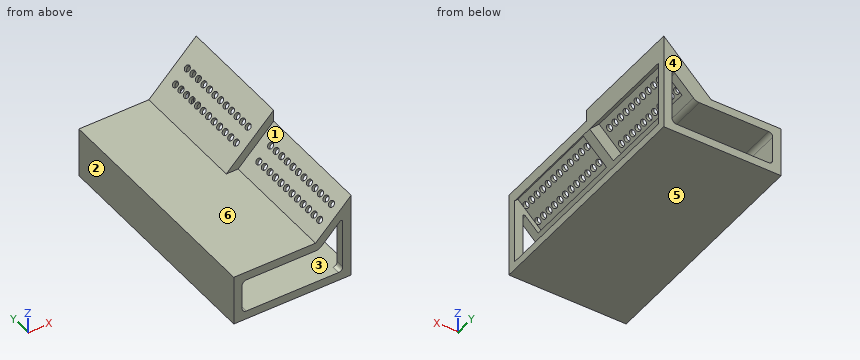
from build123d import *

# Parameters (mm, degrees)
F1_DEPTH  = 70
F3_DEPTH  = 65
F5_DEPTH  = 70
F6_R      = 2.5
F7_R      = 5
F8_R      = 1
F9_R      = 1.875
F10_DEPTH = 41.214203
F11_W     = 61.875
F11_H     = 20
F12_DEPTH = 3
F13_R     = 1.875
F14_DEPTH = 8


with BuildPart() as f1:
    # F0 (on Front) → F1 (new body, symmetric)
    with BuildSketch(Plane.XZ):
        Polygon((-35, 30), (-35, 0), (35, 0), (35, 30), (35, 51.213203), (13.786797, 30), align=None)
        Polygon((30, 5), (-30, 5), (-30, 25), (15.857864, 25), (30, 39.142136), (30, 30), align=None, mode=Mode.SUBTRACT)
    extrude(amount=F1_DEPTH, both=True)

    # F2 (on Front) → F3 (cut, symmetric)
    with BuildSketch(Plane.XZ):
        Polygon((35, 44.142136), (30, 39.142136), (30, 5), (35, 5), align=None)
    extrude(amount=F3_DEPTH, both=True, mode=Mode.SUBTRACT)

    # F4 (on face) → F5 (join)
    with BuildSketch(Plane(origin=(0, 70, 0), x_dir=(-1, 0, 0), z_dir=(0, 1, 0))):
        Polygon((-13.786797, 30), (-6.715729, 30), (-35, 58.284271), (-35, 51.213203), align=None)
    extrude(amount=-F5_DEPTH)

    # F6
    f6_edges = [f1.edges().sort_by_distance(p)[0] for p in [
        (-30, 0, 5),
        (-30, 0, 25),
        (30, 67.5, 5),
        (30, -67.5, 5),
    ]]
    fillet(f6_edges, radius=F6_R)

    # F7
    f7_edges = [f1.edges().sort_by_distance(p)[0] for p in [
        (15.857864, 0, 25),
    ]]
    fillet(f7_edges, radius=F7_R)

    # F8
    f8_edges = [f1.edges().sort_by_distance(p)[0] for p in [
        (30, 67.5, 39.142136),
        (30, -67.5, 39.142136),
    ]]
    fillet(f8_edges, radius=F8_R)

    # F9 (on face) → F10 (cut, through all)
    with BuildSketch(Plane(origin=(-11.642136, 0, 11.642136), x_dir=(0, -1, 0), z_dir=(-0.707107, 0, 0.707107))):
        with Locations((-62, 50.961941)):
            Circle(F9_R)
        with Locations((-57, 50.961941)):
            Circle(F9_R)
        with Locations((-52, 50.961941)):
            Circle(F9_R)
        with Locations((-47, 50.961941)):
            Circle(F9_R)
        with Locations((-42, 50.961941)):
            Circle(F9_R)
        with Locations((-37, 50.961941)):
            Circle(F9_R)
        with Locations((-32, 50.961941)):
            Circle(F9_R)
        with Locations((-27, 50.961941)):
            Circle(F9_R)
        with Locations((-22, 50.961941)):
            Circle(F9_R)
        with Locations((-17, 50.961941)):
            Circle(F9_R)
        with Locations((-12, 50.961941)):
            Circle(F9_R)
        with Locations((-7, 50.961941)):
            Circle(F9_R)
        with Locations((8, 50.961941)):
            Circle(F9_R)
        with Locations((13, 50.961941)):
            Circle(F9_R)
        with Locations((18, 50.961941)):
            Circle(F9_R)
        with Locations((23, 50.961941)):
            Circle(F9_R)
        with Locations((28, 50.961941)):
            Circle(F9_R)
        with Locations((33, 50.961941)):
            Circle(F9_R)
        with Locations((38, 50.961941)):
            Circle(F9_R)
        with Locations((43, 50.961941)):
            Circle(F9_R)
        with Locations((48, 50.961941)):
            Circle(F9_R)
        with Locations((53, 50.961941)):
            Circle(F9_R)
        with Locations((58, 50.961941)):
            Circle(F9_R)
        with Locations((63, 50.961941)):
            Circle(F9_R)
        with Locations((-62, 40.961941)):
            Circle(F9_R)
        with Locations((-57, 40.961941)):
            Circle(F9_R)
        with Locations((-52, 40.961941)):
            Circle(F9_R)
        with Locations((-47, 40.961941)):
            Circle(F9_R)
        with Locations((-42, 40.961941)):
            Circle(F9_R)
        with Locations((-37, 40.961941)):
            Circle(F9_R)
        with Locations((-32, 40.961941)):
            Circle(F9_R)
        with Locations((-27, 40.961941)):
            Circle(F9_R)
        with Locations((-22, 40.961941)):
            Circle(F9_R)
        with Locations((-17, 40.961941)):
            Circle(F9_R)
        with Locations((-12, 40.961941)):
            Circle(F9_R)
        with Locations((-7, 40.961941)):
            Circle(F9_R)
        with Locations((8, 40.961941)):
            Circle(F9_R)
        with Locations((13, 40.961941)):
            Circle(F9_R)
        with Locations((18, 40.961941)):
            Circle(F9_R)
        with Locations((23, 40.961941)):
            Circle(F9_R)
        with Locations((28, 40.961941)):
            Circle(F9_R)
        with Locations((33, 40.961941)):
            Circle(F9_R)
        with Locations((38, 40.961941)):
            Circle(F9_R)
        with Locations((43, 40.961941)):
            Circle(F9_R)
        with Locations((48, 40.961941)):
            Circle(F9_R)
        with Locations((53, 40.961941)):
            Circle(F9_R)
        with Locations((58, 40.961941)):
            Circle(F9_R)
        with Locations((63, 40.961941)):
            Circle(F9_R)
    extrude(amount=-F10_DEPTH, mode=Mode.SUBTRACT)

    # F11 (on face) → F12 (cut)
    with BuildSketch(Plane(origin=(-4.571068, 0, 4.571068), x_dir=(0, 1, 0), z_dir=(0.707107, 0, -0.707107))):
        with Locations((-34.0625, 45.961941)):
            Rectangle(F11_W, F11_H)
    extrude(amount=-F12_DEPTH, mode=Mode.SUBTRACT)

    # F13 (on face) → F14 (cut)
    with BuildSketch(Plane(origin=(-4.571068, 0, 4.571068), x_dir=(0, 1, 0), z_dir=(0.707107, 0, -0.707107))):
        Polygon((65, 55.961941), (3, 55.961941), (3, 35.961941), (65, 35.961941), (65, 46.47666), align=None)
        with Locations((7, 40.961941)):
            Circle(F13_R, mode=Mode.SUBTRACT)
        with Locations((12, 40.961941)):
            Circle(F13_R, mode=Mode.SUBTRACT)
        with Locations((17, 40.961941)):
            Circle(F13_R, mode=Mode.SUBTRACT)
        with Locations((22, 40.961941)):
            Circle(F13_R, mode=Mode.SUBTRACT)
        with Locations((27, 40.961941)):
            Circle(F13_R, mode=Mode.SUBTRACT)
        with Locations((32, 40.961941)):
            Circle(F13_R, mode=Mode.SUBTRACT)
        with Locations((37, 40.961941)):
            Circle(F13_R, mode=Mode.SUBTRACT)
        with Locations((42, 40.961941)):
            Circle(F13_R, mode=Mode.SUBTRACT)
        with Locations((47, 40.961941)):
            Circle(F13_R, mode=Mode.SUBTRACT)
        with Locations((52, 40.961941)):
            Circle(F13_R, mode=Mode.SUBTRACT)
        with Locations((57, 40.961941)):
            Circle(F13_R, mode=Mode.SUBTRACT)
        with Locations((62, 40.961941)):
            Circle(F13_R, mode=Mode.SUBTRACT)
        with Locations((7, 50.961941)):
            Circle(F13_R, mode=Mode.SUBTRACT)
        with Locations((12, 50.961941)):
            Circle(F13_R, mode=Mode.SUBTRACT)
        with Locations((17, 50.961941)):
            Circle(F13_R, mode=Mode.SUBTRACT)
        with Locations((22, 50.961941)):
            Circle(F13_R, mode=Mode.SUBTRACT)
        with Locations((27, 50.961941)):
            Circle(F13_R, mode=Mode.SUBTRACT)
        with Locations((32, 50.961941)):
            Circle(F13_R, mode=Mode.SUBTRACT)
        with Locations((37, 50.961941)):
            Circle(F13_R, mode=Mode.SUBTRACT)
        with Locations((42, 50.961941)):
            Circle(F13_R, mode=Mode.SUBTRACT)
        with Locations((47, 50.961941)):
            Circle(F13_R, mode=Mode.SUBTRACT)
        with Locations((52, 50.961941)):
            Circle(F13_R, mode=Mode.SUBTRACT)
        with Locations((57, 50.961941)):
            Circle(F13_R, mode=Mode.SUBTRACT)
        with Locations((62, 50.961941)):
            Circle(F13_R, mode=Mode.SUBTRACT)
    extrude(amount=-F14_DEPTH, mode=Mode.SUBTRACT)


solid = f1.part
Work out the finished part from the listing and answer in its coordinate system (mm). Face numbers are marked on the shaded views. A direction names the side the tool comes from. Coordinates: 2 decimals unless noted, no trailing zeros. Write each loop counter-clockwise with the first axis right and the second up, starting at its lowest first coordinate (ties: lowest second). Pieces come first, ordered by that corner, then holes. Notation, with made-up numbers: M 22,24.5 L 53,24.5 A19 ccw 53,57.5 Z; hole C -28.5,-39 d6. An arc over 180 degrees is marked long. Use one line per item in the form item = value. Start each with the question number.
1. Each of these flat-tipped pins is pushed along its axis until it touches: P1, Ø12, axis at x = 15, y = 41, coming from the +Z side; P2, Ø3, axis at x = -22, y = 32, coming from the +Z side; P3, Ø24.5, axis at x = -2, y = 23, coming from the +Z side. Where does it stop, or does it pass through?
2. Straight lines are drawn through the part: probe 1 along Y at (x, z) = (28.5, 45.5); probe 2 along Z at (x, y) = (-3, -38); probe 3 along X at (y, z) = (25, 14). For each, find the intervals that lie inside material, in ascending order. Write a range as from..to.
3. The part is cut by section A-A (z = 11). Give the vertices of the cut face in (x, y), plus the area to 3 significant figures.
4. The mould has two halves that part along Z. Classify the marked faces 3, 4, 5 and 6: released by +Z, released by -Z, zero draft, split by the parting line, or undercut.
5. A tool of negligible diameter and unlimited length cuts with its end or side. For the marked faces 1 and 2, from which of +Z, -Z, +X, -X, +Y, -Y can it reach the whole face along a straight path? Write none if from no direction.
6. The part is cut by section B-B (x = -7.5). Give the vertices of the cut face in (y, z).
Evaluation:
q1.P1 = 44.28
q1.P2 = 30
q1.P3 = 33.53
q2.probe_1 = 0..3, 65..70
q2.probe_2 = 0..5, 25..30
q2.probe_3 = -35..-30
q3.outline = M -35,-70 L -30,-70 L -30,70 L -35,70 Z; M 30,-70 L 35,-70 L 35,-65 L 30,-65 Z; M 30,65 L 35,65 L 35,70 L 30,70 Z
q3.area = 750 mm^2
q4.face_3 = undercut
q4.face_4 = zero draft
q4.face_5 = released by -Z
q4.face_6 = released by +Z
q5.face_1 = +Z, -X, -Y
q5.face_2 = +Z, -Z, -X, +Y, -Y
q6.outline = M -70,0 L 70,0 L 70,5 L -70,5 Z; M -70,25 L 70,25 L 70,30 L -70,30 Z
